Geometry check sheet. Reference: the model listing, model coordinates, mm. A direction names the side the tool comes from. Round coordinates to 2 decimals unless told otherwise and drop trailing zeros. Write each loop counter-clockwise with the first axis right and the second up, starting at its lowest first coordinate (ties: lowest second). Pieces come first, ordered by that corner, then holes.
Item 1: Depth check by flat-ended pin: P1, Ø1.3, axis at y = 3, z = 3.75, coming from the -X side; P2, Ø0.6, axis at y = 2.5, z = 27.5, coming from the -X side; P3, Ø0.6, axis at y = 3, z = 51.5, coming from the -X side. Enter the tip coordinate at first touch or a pass-through.
Item 2: Scan lines: probe 1 along Y at (x, z) = (-15.5, 3.75); probe 2 along Y at (x, z) = (-12.05, 51.75); probe 3 along Z at (x, y) = (-11.75, 2.5). Record each from-to range of solid material in increasing order.
Item 3: Access from +Z, -Z, +X, -X, +Y, -Y to the whole of each face (thin tool, end or side, straight path). Record for faces 1 (the face through (-1.5, 0.5, 28.1)), 2 (the face through (-18.4, 2, 27)), 3 (the face through (-15.935, 3.3, 52.704)).
Item 4: Draft check along Y on faces 4 (the face through (-9.07, 4.4, 54.93)), 5 (the face through (-12.386, 2.694, 27.011)), 6 (the face through (0, 2, 27)), 7 (the face through (-11, 0, 27)). Enter one of: pulls with the +Y half, pulls with the -Y half, needs draft (parallel to the pull), parting line crosses it, or undercut.
Item 5: Cross-section at A-A (z = 37). Enter the section's corners in (x, y).
from build123d import *

# Parameters (mm, degrees)
SKETCH1_W                       = 18.4
SKETCH1_H                       = 5
BOSS_EXTRUDE1_DEPTH             = 55.5
SKETCH2_W                       = 2.5
SKETCH2_H                       = 1
CUT_EXTRUDE1_DEPTH              = 56.5
M2X0_4_TAPPED_HOLE1_D           = 1.6
M2X0_4_TAPPED_HOLE1_DEPTH       = 7
M2X0_4_TAPPED_HOLE1_CBORE_D     = 2
M2X0_4_TAPPED_HOLE1_CBORE_DEPTH = 5
M2X0_4_TAPPED_HOLE1_TIP         = 0.480688495
FILLET1_R                       = 2


with BuildPart() as part:
    # Sketch1 → Boss-Extrude1 (new body)
    with BuildSketch(Plane.XY):
        with Locations((-9.2, 2.5)):
            Rectangle(SKETCH1_W, SKETCH1_H)
    extrude(amount=BOSS_EXTRUDE1_DEPTH)

    # Sketch2 → Cut-Extrude1 (cut, through all)
    with BuildSketch(Plane.XY.offset(55.5)):
        with Locations((-2.75, 0.5)):
            Rectangle(SKETCH2_W, SKETCH2_H)
    extrude(amount=-CUT_EXTRUDE1_DEPTH, mode=Mode.SUBTRACT)

    # M2x0.4 Tapped Hole1
    with Locations(Plane.ZY.offset(18.4)):
        with Locations((51.75, 3), (27.75, 3), (3.75, 3)):
            CounterBoreHole(M2X0_4_TAPPED_HOLE1_D / 2, M2X0_4_TAPPED_HOLE1_CBORE_D / 2, M2X0_4_TAPPED_HOLE1_CBORE_DEPTH, depth=M2X0_4_TAPPED_HOLE1_DEPTH)
            with Locations((0, 0, -(M2X0_4_TAPPED_HOLE1_DEPTH + M2X0_4_TAPPED_HOLE1_TIP / 2))):  # 118° drill point
                Cone(0, M2X0_4_TAPPED_HOLE1_D / 2, M2X0_4_TAPPED_HOLE1_TIP, mode=Mode.SUBTRACT)

    # Fillet1
    fillet1_edges = [part.edges().sort_by_distance(p)[0] for p in [
        (-9.2, 5, 0),
        (-9.2, 5, 55.5),
    ]]
    fillet(fillet1_edges, radius=FILLET1_R)


solid = part.part
Resolved:
1. P1: stops at x = -11.31
1. P2: stops at x = -13.4
1. P3: stops at x = -11.25
2. probe 1: y = 0 to 2, 4 to 5
2. probe 2: y = 0 to 2.2, 3.8 to 5
2. probe 3: z = 0 to 3.13, 4.37 to 27.13, 28.37 to 51.13, 52.37 to 55.5
3. face 1: +Z, -Z, -Y
3. face 2: +Z, -Z, -X, +Y, -Y
3. face 3: -X
4. face 4: pulls with the +Y half
4. face 5: undercut
4. face 6: needs draft
4. face 7: pulls with the -Y half
5. outline: (-18.4, 0) - (-4, 0) - (-4, 1) - (-1.5, 1) - (-1.5, 0) - (0, 0) - (0, 5) - (-18.4, 5) - close
